Geometry: final body of the model. Coordinates: model frame, mm. Face numbers are marked on the shaded views. A direction names the side the tool comes from. Give positions to 0.01 mm unless a question says otherwise; leave off trailing zeros. Loops run counter-clockwise (first coordinate to the right, second up) from the corner with the lowest first, then second, coordinate; pieces in that order, holes last. Notation, with made-up numbers: (59.25, -6.75) - (74.25, -6.75) arc R36 cw to (74.25, 31.25) - close; hole circle Ø9 at (-5, 83). An arc over 180 degrees is marked (long way). Answer in a Markdown table with one row per item.
from build123d import *

# Parameters (mm, degrees)
SKETCH_1_R          = 2.1
SKETCH_1_R_2        = 4
SKETCH_1_R_3        = 11
EXTRUDE_1_DEPTH     = 3
SKETCH_3_R          = 1
SKETCH_3_R_2        = 2.1
CUT_EXTRUDE_1_DEPTH = 99.947101842
CHAMFER_2_SIZE      = 4
CHAMFER_3_SIZE      = 10
CHAMFER_3_SIZE2     = 7.354021529
SKETCH_4_W          = 7.6
SKETCH_4_H          = 9.2
CUT_EXTRUDE_2_DEPTH = 97.00692173
FILLET_1_R          = 2
SKETCH_5_R          = 2.1
CUT_EXTRUDE_3_DEPTH = 97.00692173
CHAMFER_1_SIZE      = 2


with BuildPart() as part:
    # 草图1 → 凸台-拉伸1 (new, symmetric)
    with BuildSketch(Plane.XY):
        with BuildLine():
            Line((-55, 82.03370626), (-55, -2.96629374))
            Line((-55, -2.96629374), (-35, -2.96629374))
            Line((-35, -2.96629374), (-32.567908633, -10.505776978))
            ThreePointArc((-32.567908633, -10.505776978), (-3.332171442, -34.057842799), (29.91406589, -16.618925494))
            Line((29.91406589, -16.618925494), (51.767997793, 22.718151931))
            Line((51.767997793, 22.718151931), (-55, 82.03370626))
        make_face()
        with Locations((29, 0)):
            Circle(SKETCH_1_R, mode=Mode.SUBTRACT)
        with Locations((-14.5, -25.11473671)):
            Circle(SKETCH_1_R, mode=Mode.SUBTRACT)
        with Locations((-14.5, 25.11473671)):
            Circle(SKETCH_1_R, mode=Mode.SUBTRACT)
        with Locations((-9.625, 16.670989023)):
            Circle(SKETCH_1_R_2, mode=Mode.SUBTRACT)
        Circle(SKETCH_1_R_3, mode=Mode.SUBTRACT)
    extrude(amount=EXTRUDE_1_DEPTH, both=True)

    # 草图3 → 切除-拉伸1 (cut, through all)
    with BuildSketch(Plane.XY.offset(3)):
        with Locations((-35.951708618, -3.273296519)):
            Circle(SKETCH_3_R)
        with Locations((-45, 7.03370626)):
            Circle(SKETCH_3_R_2)
        with Locations((-45, 57.03370626)):
            Circle(SKETCH_3_R_2)
    extrude(amount=-CUT_EXTRUDE_1_DEPTH, mode=Mode.SUBTRACT)

    # 倒角2
    chamfer_2_edges = [part.edges().sort_by_distance(p)[0] for p in [
        (51.767997793, 22.718151931, 0),
        (-55, -2.96629374, 0),
    ]]
    chamfer(chamfer_2_edges, length=CHAMFER_2_SIZE)

    # 倒角3
    chamfer_3_edges = [part.edges().sort_by_distance(p)[0] for p in [
        (-55, 82.03370626, 0),
    ]]
    chamfer_3_side = [part.faces().sort_by_distance(p)[0] for p in [
        (-55, 41.53370626, 0),
    ]]
    chamfer(chamfer_3_edges, length=CHAMFER_3_SIZE, length2=CHAMFER_3_SIZE2, reference=chamfer_3_side[0])

    # 草图4 → 切除-拉伸2 (cut, through all)
    with BuildSketch(Plane.XY.offset(3)):
        with Locations((-18.5, 0)):
            Rectangle(SKETCH_4_W, SKETCH_4_H)
    extrude(amount=-CUT_EXTRUDE_2_DEPTH, mode=Mode.SUBTRACT)

    # 圆角1
    fillet_1_edges = [part.edges().sort_by_distance(p)[0] for p in [
        (-14.7, 4.6, 0),
        (-14.7, -4.6, 0),
        (-22.3, -4.6, 0),
        (-22.3, 4.6, 0),
    ]]
    fillet(fillet_1_edges, radius=FILLET_1_R)

    # 草图5 → 切除-拉伸3 (cut, through all)
    with BuildSketch(Plane.XY.offset(3)):
        with Locations((-5.537868087, 43.115155041)):
            Circle(SKETCH_5_R)
        with Locations((38.16999572, 18.833008482)):
            Circle(SKETCH_5_R)
    extrude(amount=-CUT_EXTRUDE_3_DEPTH, mode=Mode.SUBTRACT)

    # 倒角1
    chamfer_1_edges = [part.edges().sort_by_distance(p)[0] for p in [
        (-7.637868087, 43.115155041, -3),
        (36.06999572, 18.833008482, -3),
        (-47.1, 7.03370626, -3),
        (-47.1, 57.03370626, -3),
    ]]
    chamfer(chamfer_1_edges, length=CHAMFER_1_SIZE)


solid = part.part
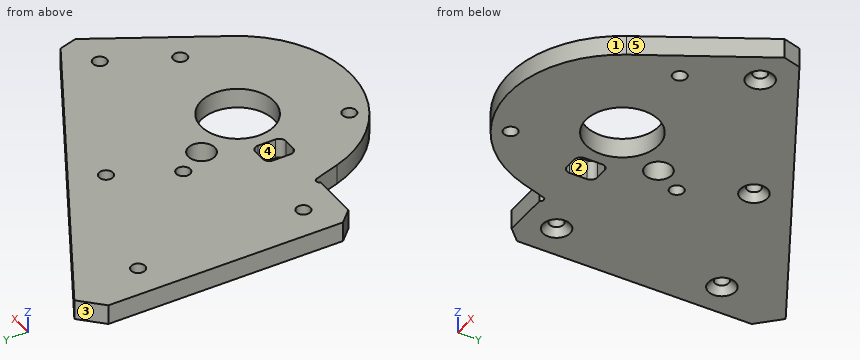
Q1. Cut plane A-A (x = 0). Output: boundary loops of the cut face in (y, z), and give its area (3 significant figures).
Check values:
| item | result |
|---|---|
| outline | (-34.22, -3) - (-11, -3) - (-11, 3) - (-34.22, 3) - close; (11, -3) - (51.48, -3) - (51.48, 3) - (11, 3) - close |
| area | 382 mm² |
Q2. Reachability of the marked faces 1 and 2 from +Z, -Z, +X, -X, +Y, -Y: full face, straight path, thin tool, end or side. Return the list, or none.
Check values:
| item | result |
|---|---|
| face 1 | +Z, -Z, -Y |
| face 2 | +Z, -Z |
Q3. Draft query along X for the marked faces 3, 4 and 5. Return one class per face: pulls with the +X half, pulls with the -X half, needs draft (parallel to the pull), parting line crosses it, or undercut.
Check values:
| item | result |
|---|---|
| face 3 | pulls with the -X half |
| face 4 | undercut |
| face 5 | pulls with the +X half |
Q4. Cut plane B-B (z = 0.75). Give the number of separate pieces and of enclosed holes in the cut face, and give its area (3 significant figures).
Check values:
| item | result |
|---|---|
| separate pieces | 1 |
| enclosed holes | 10 |
| area | 6,740 mm² |
Q5. First-contact query: pin 1 (3 mm diameter, centred on x = -46.5, z = -0.5, fed in from -Y); pin 2 (5.5 mm diameter, centred on x = -14.5, y = 25.11, fed in from -Z); pin 3 (2 mm diameter, centred on y = -13.5, z = -2, fed in from +X); pin 4 (3 mm diameter, centred on x = -18.5, z = -0.5, fed in from -Y). Flat tips, straight axial feed; report the tip coordinate or a pass-through.
Check values:
| item | result |
|---|---|
| pin 1 | y = -2.97 |
| pin 2 | z = -3 |
| pin 3 | x = 32.2 |
| pin 4 | y = -29.7 |
Q6. Cut plane D-D (y = 31). Output: boundary loops of the cut face in (x, z).
Check values:
| item | result |
|---|---|
| outline | (-55, -3) - (36.86, -3) - (36.86, 3) - (-55, 3) - close |
Q7. Material intervals for line 1 along X through (y, z) = (19.5, 2.75); line 2 along Y through (x, z) = (-45, 2.15); line 3 along Y through (x, z) = (-9, 2), sorted ascending.
Check values:
| item | result |
|---|---|
| line 1 | -55 to -12.45, -6.8 to 36.18, 40.16 to 49.75 |
| line 2 | -2.97 to 4.93, 9.13 to 54.93, 59.13 to 76.48 |
| line 3 | -33.02 to -6.32, 6.32 to 12.72, 20.62 to 56.48 |
Q8. Cut plane C-C (x = 21.5). Output: boundary loops of the cut face in (y, z), and give its area (3 significant figures).
Check values:
| item | result |
|---|---|
| outline | (-26.62, -3) - (39.53, -3) - (39.53, 3) - (-26.62, 3) - close |
| area | 397 mm² |
